```python
from build123d import *

# Parameters (mm, degrees)
SKETCH1_W                = 82.55
SKETCH1_H                = 56.4134
BOSS_EXTRUDE1_DEPTH      = 8.1534
CUT_EXTRUDE1_START       = -88.085249325
CUT_EXTRUDE1_OUTLINE_W   = 8.1534
CUT_EXTRUDE1_OUTLINE_H   = 8.1534
CUT_EXTRUDE1_DEPTH       = 16.51
CUT_EXTRUDE1_START_2     = -55.065249325
CUT_EXTRUDE1_2_OUTLINE_W = 8.1534
CUT_EXTRUDE1_2_OUTLINE_H = 8.1534
CUT_EXTRUDE1_2_DEPTH     = 16.51
CUT_EXTRUDE1_START_3     = -22.045249325
CUT_EXTRUDE1_3_OUTLINE_W = 8.1534
CUT_EXTRUDE1_3_OUTLINE_H = 8.1534
CUT_EXTRUDE1_3_DEPTH     = 16.51
SKETCH3_W                = 8.1534
SKETCH3_H                = 12.065106948
CUT_EXTRUDE2_DEPTH       = 99.056076844
SKETCH4_R                = 18.542
CUT_EXTRUDE3_DEPTH       = 99.056076844


# Read off the part's stored shape, not the designer's step: Cut-Extrude1
with BuildPart() as part:
    # Sketch1 → Boss-Extrude1 (new body)
    with BuildSketch(Plane.XY):
        with Locations((-46.810249325, -14.095842782)):
            Rectangle(SKETCH1_W, SKETCH1_H)
    extrude(amount=BOSS_EXTRUDE1_DEPTH)

    # Cut-Extrude1 outline → Cut-Extrude1 (cut)
    with BuildSketch(Plane.YZ.offset(CUT_EXTRUDE1_START)):
        with Locations((10.034157218, 4.0767)):
            Rectangle(CUT_EXTRUDE1_OUTLINE_W, CUT_EXTRUDE1_OUTLINE_H)
    extrude(amount=CUT_EXTRUDE1_DEPTH, mode=Mode.SUBTRACT)

    # Cut-Extrude1 2 outline → Cut-Extrude1 2 (cut)
    with BuildSketch(Plane.YZ.offset(CUT_EXTRUDE1_START_2)):
        with Locations((10.034157218, 4.0767)):
            Rectangle(CUT_EXTRUDE1_2_OUTLINE_W, CUT_EXTRUDE1_2_OUTLINE_H)
    extrude(amount=CUT_EXTRUDE1_2_DEPTH, mode=Mode.SUBTRACT)

    # Cut-Extrude1 3 outline → Cut-Extrude1 3 (cut)
    with BuildSketch(Plane.YZ.offset(CUT_EXTRUDE1_START_3)):
        with Locations((10.034157218, 4.0767)):
            Rectangle(CUT_EXTRUDE1_3_OUTLINE_W, CUT_EXTRUDE1_3_OUTLINE_H)
    extrude(amount=CUT_EXTRUDE1_3_DEPTH, mode=Mode.SUBTRACT)

    # Sketch3 → Cut-Extrude2 (cut, through all)
    with BuildSketch(Plane.XY.offset(8.1534)):
        with Locations((-84.008549325, -36.269989308)):
            Rectangle(SKETCH3_W, SKETCH3_H)
        with Locations((-84.008549325, -12.139775411)):
            Rectangle(SKETCH3_W, SKETCH3_H)
        with Locations((-9.611949325, -36.269989308)):
            Rectangle(SKETCH3_W, SKETCH3_H)
        with Locations((-9.611949325, -12.139775411)):
            Rectangle(SKETCH3_W, SKETCH3_H)
    extrude(amount=-CUT_EXTRUDE2_DEPTH, mode=Mode.SUBTRACT)

    # Sketch4 → Cut-Extrude3 (cut, through all)
    with BuildSketch(Plane(origin=(0, 0, 0), x_dir=(-1, 0, 0), z_dir=(0, 0, -1))):
        with Locations((46.810249325, -13.092542782)):
            Circle(SKETCH4_R)
    extrude(amount=-CUT_EXTRUDE3_DEPTH, mode=Mode.SUBTRACT)


solid = part.part
```
Input: part model. Units: mm. Frame: model coordinates. A direction names the side the tool comes from. Coordinates: 2 decimals unless noted, no trailing zeros. Loops run counter-clockwise (first coordinate to the right, second up) from the corner with the lowest first, then second, coordinate; pieces in that order, holes last. Notation, with made-up numbers: (17, -11) - (41, -11) arc R25 cw to (41, 11) - close; hole circle Ø8 at (32.5, 5). An arc over 180 degrees is marked (long way). Answer in a Markdown table with one row per item.
(1) Cut plane B-B on x = -81. Output: boundary loops of the cut face in (y, z).
Model answer:
| item | result |
|---|---|
| outline | (-30.24, 0) - (-18.17, 0) - (-18.17, 8.15) - (-30.24, 8.15) - close; (-6.11, 0) - (5.96, 0) - (5.96, 8.15) - (-6.11, 8.15) - close |
(2) Mould query, pull axis X, two halves, no side actions, for faces 5 (the face through (-63, 14.111, 4)), 6 (the face through (-13.689, -36, 4)), 7 (the face through (-47, 5.957, 4)). Classes: pulls with the +X half, pulls with the -X half, needs draft (parallel to the pull), parting line crosses it, or undercut.
Model answer:
| item | result |
|---|---|
| face 5 | needs draft |
| face 6 | pulls with the +X half |
| face 7 | undercut |
(3) Cut plane C-C on z = 5.25. Output: boundary loops of the cut face in (x, y).
Model answer:
| item | result |
|---|---|
| outline | (-88.09, -30.24) - (-79.93, -30.24) - (-79.93, -42.3) - (-13.69, -42.3) - (-13.69, -30.24) - (-5.54, -30.24) - (-5.54, -18.17) - (-13.69, -18.17) - (-13.69, -6.11) - (-5.54, -6.11) - (-5.54, 5.96) - (-22.05, 5.96) - (-22.05, 14.11) - (-38.56, 14.11) - (-38.56, 5.96) - (-55.07, 5.96) - (-55.07, 14.11) - (-71.58, 14.11) - (-71.58, 5.96) - (-88.09, 5.96) - (-88.09, -6.11) - (-79.93, -6.11) - (-79.93, -18.17) - (-88.09, -18.17) - close; hole circle Ø37.08 at (-46.81, -13.09) |
(4) Pin query (flat end, axial travel): P1, Ø4, axis at y = -12.5, z = 1.5, coming from the +X side; P2, Ø4, axis at x = -43, z = 4, coming from the +Y side; P3, Ø3, axis at y = -16.5, z = 7, coming from the -X side. Return the tip coordinate at first contact, or that it passes through.
Model answer:
| item | result |
|---|---|
| P1 | stops at x = -13.69 |
| P2 | stops at y = 5.96 |
| P3 | stops at x = -79.93 |
(5) Material intervals for L1, parallel to X at y = 9, z = 7; L2, parallel to Y at x = -11, z = 1.25; L3, parallel to X at y = -13, z = 4.5, sorted ascending. Write a range as from..to.
Model answer:
| item | result |
|---|---|
| L1 | x = -71.58..-55.07, -38.56..-22.05 |
| L2 | y = -30.24..-18.17, -6.11..5.96 |
| L3 | x = -79.93..-65.35, -28.27..-13.69 |
(6) Set-up query: faces 1 (the face through (-38.555, 10, 4)), 2 (the face through (-14, 5.957, 4)), 3 (the face through (-71.575, 10, 4)), 4 (the face through (-10, -30.237, 4)). Return all of +Z, -Z, +X, -X, +Y, -Y with unobstructed straight access to the full face (end or side cutting, diameter ignored); none if empty.
Model answer:
| item | result |
|---|---|
| face 1 | +Z, -Z, +Y |
| face 2 | +Z, -Z, +X, +Y |
| face 3 | +Z, -Z, -X, +Y |
| face 4 | +Z, -Z, +X, -Y |
(7) Cut plane A-A on y = 7. Output: boundary loops of the cut face in (x, z).
Model answer:
| item | result |
|---|---|
| outline | (-71.58, 0) - (-55.07, 0) - (-55.07, 8.15) - (-71.58, 8.15) - close; (-38.56, 0) - (-22.05, 0) - (-22.05, 8.15) - (-38.56, 8.15) - close |
(8) Cut plane D-D on y = -37. Output: boundary loops of the cut face in (x, z).
Model answer:
| item | result |
|---|---|
| outline | (-79.93, 0) - (-13.69, 0) - (-13.69, 8.15) - (-79.93, 8.15) - close |
